Design review of the part shown in the three views and the two pictorial views. Dimensions are in mm from the part's minimum x, y and z. Coordinates: 2 decimals unless noted, no trailing zeros. Loops run counter-clockwise (first coordinate to the right, second up) from the corner with the lowest first, then second, coordinate; pieces in that order, holes last. Notation, with made-up numbers: M 49.25,86 L 79.25,86 A13 ccw 79.25,90 Z; hole C 12.5,5.25 d1. An arc over 180 degrees is marked long. Answer as a JSON object with one key per item and string values. Group by question number.
Item 1: Add section B-B (y = 0.5). State the section outline as (x, z) points (3 decimals).
Item 2: Insertion check: pin 1 (0.6 mm diameter, centred on x = 0.5, z = 2, fed in from +Y); pin 2 (6 mm diameter, centred on y = 10, z = 5, fed in from +X); pin 3 (1.5 mm diameter, centred on x = 1.5, y = 14, fed in from -Z); pin 4 (1.5 mm diameter, centred on y = 16, z = 7, fed in from -X). Each pin has a flat end and moves straight along its axis. Give the tip position at first contact, or say it passes through.
Item 3: Wall thickness on L1, parallel to X at y = 0.5, z = 2 (3 decimals); L2, parallel to Y at x = 4.5, z = 1.25; L3, parallel to Y at x = 2.2, z = 4.5: over which ranges is each line inside the solid? List them lowest first. Write a range as from..to.
Item 4: Add section C-C (z = 4). Count the separate pieces of the cut face and the enclosed holes in it, then the cut area to 3 significant figures.
Item 5: Add section A-A (y = 8). State the section outline as (x, z) points (3 decimals), then the cut area to 3 significant figures.
Item 6: Add section D-D (y = 10.5). State the section outline as (x, z) points, then the cut area to 3 significant figures.
Item 7: Mouldability with a two-part tool opening along Y and no side actions: class the marked faces 1, 2 and 3 as +Y half, -Y half, draft (parallel to the pull), parting line (faces both ways), or undercut.
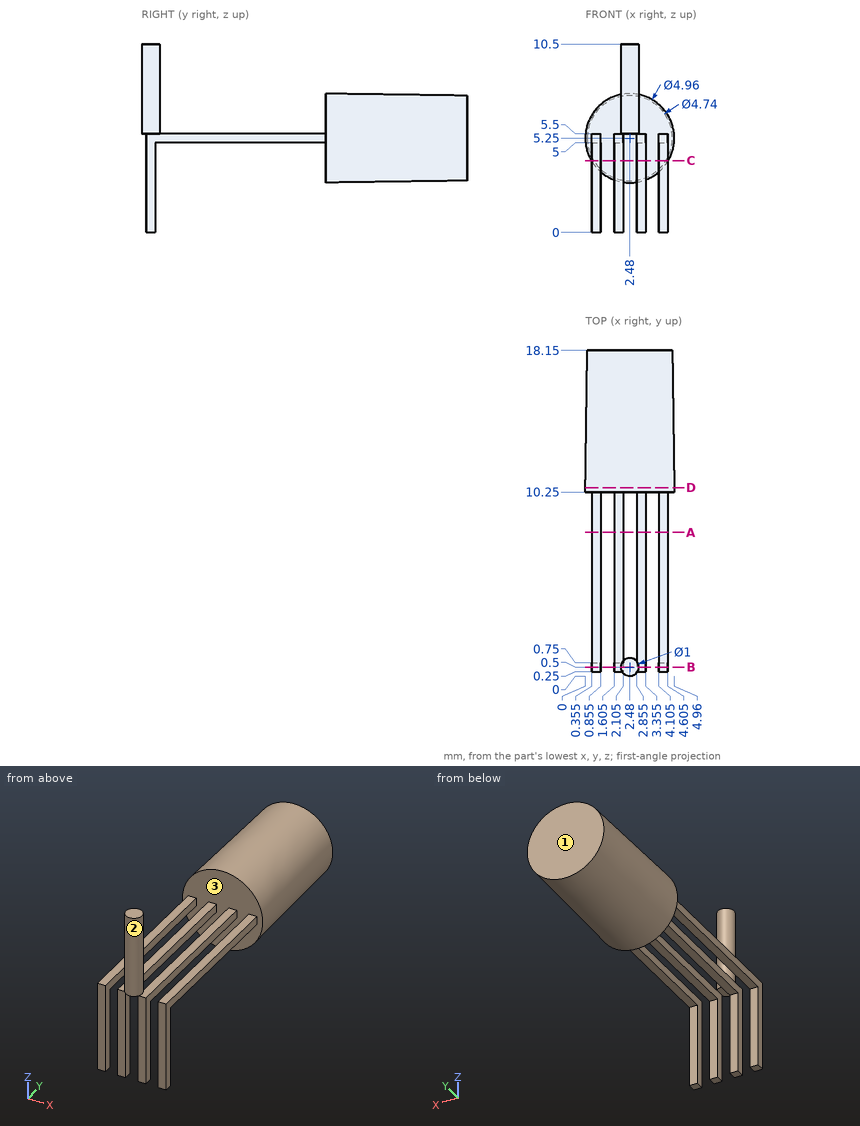
From the geometry:
{
 "1": {"outline": "M 0.355,0 L 0.855,0 L 0.855,5.5 L 0.355,5.5 Z; M 1.605,0 L 2.105,0 L 2.105,5.5 L 2.855,5.5 L 2.855,0 L 3.355,0 L 3.355,5.5 L 2.98,5.5 L 2.98,10.5 L 1.98,10.5 L 1.98,5.5 L 1.605,5.5 Z; M 4.105,0 L 4.605,0 L 4.605,5.5 L 4.105,5.5 Z"},
 "2": {"pin 1": "stops at y = 0.75", "pin 2": "stops at x = 4.96", "pin 3": "stops at z = 2.83", "pin 4": "stops at x = 0.3"},
 "3": {"L1": "x = 0.355..0.855, 1.605..2.105, 2.855..3.355, 4.105..4.605", "L2": "y = 0.25..0.75", "L3": "y = 10.25..18.15"},
 "4": {"separate pieces": "5", "enclosed holes": "0", "area": "33.8 mm²"},
 "5": {"outline": "M 0.355,5 L 0.855,5 L 0.855,5.5 L 0.355,5.5 Z; M 1.605,5 L 2.105,5 L 2.105,5.5 L 1.605,5.5 Z; M 2.855,5 L 3.355,5 L 3.355,5.5 L 2.855,5.5 Z; M 4.105,5 L 4.605,5 L 4.605,5.5 L 4.105,5.5 Z", "area": "1.00 mm²"},
 "6": {"outline": "C 2.48,5.25 d4.95", "area": "19.3 mm²"},
 "7": {"face 1": "+Y half", "face 2": "undercut", "face 3": "undercut"}
}
